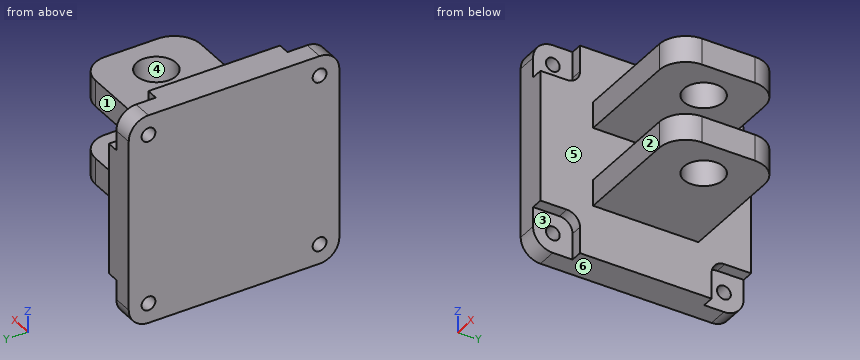
Autodesk Inventor part; units mm, degrees
ref_plane "YZ Plane" through (0, 0, 0) normal (1, 0, 0) x (0, 1, 0)
ref_plane "XZ Plane" through (0, 0, 0) normal (0, 1, 0) x (-1, 0, 0)
ref_plane "XY Plane" through (0, 0, 0) normal (0, 0, 1) x (1, 0, 0)
sketch "Skizze1" plane through (0, 0, 0) normal (0, 0, 1) x (1, 0, 0)
  line L0 (0, 80) -> (24, 80)
  line L1 (24, 80) -> (24, -80)
  line L2 (24, -80) -> (0, -80)
  line L3 (0, -80) -> (0, 80)
  line L4 (24, 40) -> (124, 40)
  line L5 (124, 40) -> (124, -40)
  line L6 (124, -40) -> (24, -40)
  line L7 (24, -40) -> (24, 40)
  point P0 (0, 0)
  point P1 (24, 0)
  point P2 (0, 0)
  point P3 (94, 0)
  point P4 (124, 0)
  dimension "d0" = 160
  dimension "d1" = 24
  dimension "d2" = 124
  dimension "d3" = 80
  dimension "d4" = 94
extrude "Extrusion1" add sketch "Skizze1" along normal mid plane 160 contours L0 L1 L2 L3
extrude "Extrusion2" add sketch "Skizze1" along normal mid plane 80 contours L4 L5 L6 L1
extrude "Extrusion3" cut sketch "Skizze1" along normal mid plane 40 contours L4 L5 L6 L1
fillet "Rundung1" radius 20 4 edges at (124, 40, 30) (124, 40, -30) (124, -40, -30) (124, -40, 30)
hole "Bohrung1" at (94, 0, 0) direction (0, 0, -1) diameter 30 end through all both
sketch "Skizze2" plane through (24, -80, 80) normal (1, 0, 0) x (0, 0, -1)
  line L0 (0, 160) -> (30, 160)
  line L1 (30, 160) -> (30, 130)
  line L2 (30, 130) -> (0, 130)
  line L3 (0, 130) -> (0, 160)
  point P0 (80, 80)
  dimension "d19" = 30
  dimension "d20" = 30
extrude "Extrusion4" cut sketch "Skizze2" against normal blind 9
pattern_circular "Runde Anordnung1" count 4 over 360 about axis through (-10, 0, 0) along (1, 0, 0) of "Extrusion4"
sketch "Skizze3" plane through (24, 50, 50) normal (1, 0, 0) x (0, 0, -1)
  line L0 (-15, 15) -> (115, 15)
  line L1 (115, 15) -> (115, -115)
  line L2 (115, -115) -> (-15, -115)
  line L3 (-15, -115) -> (-15, 15)
  line L4 (-15, 15) -> (115, -115) construction
  line L5 (115, 15) -> (-15, -115) construction
  point P0 (50, -50)
  dimension "d26" = 130
  dimension "d27" = 130
hole "Bohrung2" at (24, 65, 65) at (24, -65, 65) at (24, 65, -65) at (24, -65, -65) direction (-1, 0, 0) diameter 10.5 end through all
fillet "Rundung2" radius 15 4 edges at (7.5, 80, -80) (7.5, -80, -80) (7.5, -80, 80) (7.5, 80, 80)
fillet "Rundung3" radius 10 4 edges at (19.5, -50, 50) (19.5, -50, -50) (19.5, 50, -50) (19.5, 50, 50)
equation "\"d5\" = d0"
properties part number "Befestigungsflansch" material "Stahl AISI 4130"
Here's how the part is built. I have some questions about the finished solid (model axes, mm). Face numbers are marked on the shaded views. A direction names the side the tool comes from. Coordinates: 2 decimals unless noted, no trailing zeros. Order: outer loops, then holes, each group sorted by start corner. A loop starts at its lowest first (then second) coordinate and runs counter-clockwise, first axis right, second up. Notation, with made-up numbers: M -8.75,22 L 36.25,22 A24 cw 36.25,34 Z; hole C -13,-12.75 d3. An arc over 180 degrees is marked long. Answer as a JSON object with one key per item and string values. Group by question number.
(1) I need wall thicknesses on probe 1 along Y at (x, z) = (11, 65); probe 2 along Y at (x, z) = (94, 30.25). Which ranges of each line are inside material? Lowest first, please.
(2) Suppose I cut it at D-D, the plane x = 41. Please give me the cut outline in (y, z), then the cut area to 3 significant figures.
(3) If we mould it in two halves opening along Z, with no side actions, what happens to the marked faces 4, 5 and 6? For each: released by +Z, released by -Z, zero draft, split by the parting line, or undercut.
(4) Which directions (+Z, -Z, +X, -X, +Y, -Y) give clear straight access to the entire face, cutting with the end or side of a thin tool? Please do the marked faces 1, 2 and 3.
(5) Suppose I cut it at B-B, the plane x = 94. Please give me the cut outline in (y, z), then the cut area to 3 significant figures.
(6) For pin 1 (10 mm diameter, centred on x = 103.5, y = -34, fed in from +Z); pin 2 (22 mm diameter, centred on x = 46, z = -27.5, fed in from -Y); pin 3 (16 mm diameter, centred on x = 63, z = 31.5, fed in from +Y), each with a flat end and sliding along its axis, tell me the tip position at first contact or that it passes through.
(7) Suppose I cut it at A-A, the plane y = 0. Please give me the cut outline in (x, z).
(8) Suppose I cut it at C-C, the plane z = -29. Please give me the cut outline in (x, y), then the cut area to 3 significant figures.
Values found:
{
 "1": {"probe 1": "y = -80 to -70.25, -59.75 to 59.75, 70.25 to 80", "probe 2": "y = -40 to -15, 15 to 40"},
 "2": {"outline": "M -40,-40 L 40,-40 L 40,-20 L -40,-20 Z; M -40,20 L 40,20 L 40,40 L -40,40 Z", "area": "3,200 mm^2"},
 "3": {"face 4": "zero draft", "face 5": "undercut", "face 6": "released by -Z"},
 "4": {"face 1": "+Z, -Z, +X, +Y", "face 2": "+Z, -Z, +X, -Y", "face 3": "-Z, +X, -Y"},
 "5": {"outline": "M -40,-40 L -15,-40 L -15,-20 L -40,-20 Z; M -40,20 L -15,20 L -15,40 L -40,40 Z; M 15,-40 L 40,-40 L 40,-20 L 15,-20 Z; M 15,20 L 40,20 L 40,40 L 15,40 Z", "area": "2,000 mm^2"},
 "6": {"pin 1": "stops at z = 40", "pin 2": "stops at y = -40", "pin 3": "stops at y = 40"},
 "7": {"outline": "M 0,-80 L 24,-80 L 24,-40 L 79,-40 L 79,-20 L 24,-20 L 24,20 L 79,20 L 79,40 L 24,40 L 24,80 L 0,80 Z; M 109,-40 L 124,-40 L 124,-20 L 109,-20 Z; M 109,20 L 124,20 L 124,40 L 109,40 Z"},
 "8": {"outline": "M 0,-80 L 24,-80 L 24,-40 L 104,-40 A20 ccw 124,-20 L 124,20 A20 ccw 104,40 L 24,40 L 24,80 L 0,80 Z; hole C 94,0 d30", "area": "11,000 mm^2"}
}
